```python
from build123d import *

# Parameters (mm, degrees)
SKETCH1_R           = 10
BOSS_EXTRUDE1_DEPTH = 60
SKETCH2_R           = 7.5
BOSS_EXTRUDE2_DEPTH = 30
CHAMFER2_SIZE       = 5
SKETCH3_R           = 7.5
BOSS_EXTRUDE3_DEPTH = 20
CHAMFER3_SIZE       = 4
CHAMFER3_SIZE2      = 4.76701437
SKETCH5_W           = 6
SKETCH5_H           = 55
BOSS_EXTRUDE5_DEPTH = 12
SKETCH6_W           = 2.4
SKETCH6_H           = 10
BOSS_EXTRUDE6_DEPTH = 10
SKETCH13_W          = 6
SKETCH13_H          = 1
CUT_EXTRUDE2_DEPTH  = 10
SKETCH14_W          = 6
SKETCH14_H          = 1
CUT_EXTRUDE3_DEPTH  = 5
CHAMFER22_SIZE      = 0.5
CHAMFER22_SIZE_2    = 1.866025404
SKETCH17_W          = 1
SKETCH17_H          = 2.5
BOSS_EXTRUDE7_DEPTH = 0.5
FILLET1_R           = 1
FILLET2_R           = 5


with BuildPart() as part:
    # Sketch1 → Boss-Extrude1 (new body)
    with BuildSketch(Plane(origin=(0, 0, 0), x_dir=(1, 0, 0), z_dir=(0, 1, 0))):
        with Locations(Location((0, 0, 0), (0, 0, 90))):
            Circle(SKETCH1_R)
    extrude(amount=BOSS_EXTRUDE1_DEPTH)

    # Sketch2 → Boss-Extrude2 (add)
    with BuildSketch(Plane(origin=(0, 60, 0), x_dir=(1, 0, 0), z_dir=(0, 1, 0))):
        with Locations(Location((0, 0, 0), (0, 0, 270))):
            Circle(SKETCH2_R)
    extrude(amount=BOSS_EXTRUDE2_DEPTH)

    # Chamfer2
    # the kernel refuses this chamfer: 5 mm, written as the material it takes off along each edge
    with BuildSketch(Plane(origin=(0, 60, 0), x_dir=(0, 0, -1), z_dir=(1, 0, 0))) as chamfer2_piece_1_section:
        Polygon((10, -CHAMFER2_SIZE), (10 - CHAMFER2_SIZE, 0), (10, 0), align=None)
    chamfer2_piece_1 = revolve(axis=Axis((0, 60, 0), (0, 1, 0)), mode=Mode.PRIVATE)
    chamfer2_piece_1 = chamfer2_piece_1 - Plane(origin=(0, 56.238108378, 0), x_dir=(0, 0, 1), z_dir=(0, -1, 0)) * Cylinder(7.5, 40, mode=Mode.PRIVATE)
    add(chamfer2_piece_1, mode=Mode.SUBTRACT)

    # Sketch3 → Boss-Extrude3 (add)
    with BuildSketch(Plane(origin=(0, 90, 0), x_dir=(1, 0, 0), z_dir=(0, 1, 0))):
        with Locations(Location((0, 0, 0), (0, 0, 90))):
            Circle(SKETCH3_R)
    extrude(amount=BOSS_EXTRUDE3_DEPTH)

    # Chamfer3
    chamfer3_edges = [part.edges().sort_by_distance(p)[0] for p in [
        (0, 110, 7.5),
    ]]
    chamfer3_side = [part.faces().sort_by_distance(p)[0] for p in [
        (0, 110, 0),
    ]]
    chamfer(chamfer3_edges, length=CHAMFER3_SIZE, length2=CHAMFER3_SIZE2, reference=chamfer3_side[0])

    # Sketch5 → Boss-Extrude5 (add)
    with BuildSketch(Plane(origin=(0, 0, 0), x_dir=(0, 0, -1), z_dir=(1, 0, 0))):
        with Locations((0, 27.5)):
            Rectangle(SKETCH5_W, SKETCH5_H)
    extrude(amount=BOSS_EXTRUDE5_DEPTH)

    # Sketch6 → Boss-Extrude6 (add)
    with BuildSketch(Plane(origin=(0, 0, 0), x_dir=(0, 0, -1), z_dir=(1, 0, 0))):
        with Locations((0, 87.067071975)):
            Rectangle(SKETCH6_W, SKETCH6_H)
    extrude(amount=BOSS_EXTRUDE6_DEPTH)

    # Sketch13 → Cut-Extrude2 (cut)
    with BuildSketch(Plane(origin=(0, 110, 0), x_dir=(1, 0, 0), z_dir=(0, 1, 0))):
        Rectangle(SKETCH13_W, SKETCH13_H)
    extrude(amount=-CUT_EXTRUDE2_DEPTH, mode=Mode.SUBTRACT)

    # Sketch14 → Cut-Extrude3 (cut)
    with BuildSketch(Plane(origin=(0, 100, 0), x_dir=(1, 0, 0), z_dir=(0, 1, 0))):
        Rectangle(SKETCH14_W, SKETCH14_H)
    extrude(amount=-CUT_EXTRUDE3_DEPTH, mode=Mode.SUBTRACT)

    # Chamfer22
    # the kernel refuses this chamfer: 1.866025404, 0.5 mm, written as the material it takes off along each edge
    with BuildSketch(Plane(origin=(3, 110, 0.5), x_dir=(0.9905000388259552, 0.13751244702128432, 0), z_dir=(0, 0, -1)), Plane(origin=(-3, 110, -0.5), x_dir=(-0.9905000388259552, 0.13751244702128432, 0), z_dir=(0, 0, 1))) as chamfer22_piece_1:
        Polygon((CHAMFER22_SIZE * 0.990500038826, CHAMFER22_SIZE * 0.137512447021), (-CHAMFER22_SIZE_2 * 0.137512447005, CHAMFER22_SIZE_2 * 0.990500038712), (0, 0), align=None)
    extrude(amount=1, mode=Mode.SUBTRACT)

    # Sketch17 → Boss-Extrude7 (add)
    with BuildSketch(Plane(origin=(0, 0, 0.5), x_dir=(-1, 0, 0), z_dir=(0, 0, -1))):
        with Locations((0, 101.254046964)):
            Rectangle(SKETCH17_W, SKETCH17_H)
    extrude(amount=BOSS_EXTRUDE7_DEPTH)

    # Fillet1
    # the kernel refuses this fillet: 1 mm, written as the material it takes off along each edge
    with BuildSketch(Plane(origin=(-2.665063509, 102.504046964, 0), x_dir=(0, 0, 1), z_dir=(1, 0, 0))) as fillet1_piece_1:
        with BuildLine():
            CenterArc((1, 0.866025404), FILLET1_R, 180, 60)
            Line((0, 0.866025404), (-0.02, 0.866025404))
            Line((-0.02, 0.866025404), (-0.02, 0))
            Line((-0.02, 0), (0, -0.02))
            ThreePointArc((0, -0.02), (0.25, -0.02), (0.49, -0.017320508))
            Line((0.49, -0.017320508), (0.5, 0))
        make_face()
    extrude(amount=5.330127019, mode=Mode.SUBTRACT)

    # Fillet2
    fillet2_edges = [part.edges().sort_by_distance(p)[0] for p in [
        (3, 108.133974596, 0),
        (-3, 108.133974596, 0),
    ]]
    fillet(fillet2_edges, radius=FILLET2_R)


solid = part.part
```
Work out the finished part from the listing and answer in its coordinate system (mm). A direction names the side the tool comes from. Round coordinates to 2 decimals unless told otherwise and drop trailing zeros. Write each loop counter-clockwise with the first axis right and the second up, starting at its lowest first coordinate (ties: lowest second). Pieces come first, ordered by that corner, then holes. Notation, with made-up numbers: (28.5, 5) - (59.5, 5) arc R28 cw to (59.5, 40) - close; hole circle Ø8 at (3, 25). An arc over 180 degrees is marked (long way). Return JSON: item names as keys, results as strings. Group by question number.
Q1. The part is cut by section C-C on y = 9.5. Write down the section's boundary in (x, z), then the cut area to 3 significant figures.
Q2. The mould has two halves that part along Z. Classify faces 1 (the flat face through (1, 0, 0)), 2 (the flat face through (11, 27, -3)), 3 (the flat face through (11, 27, 3)), 4 (the flat face through (-1, 102, 0.5)): released by +Z, released by -Z, zero draft, split by the parting line, or undercut.
Q3. The part is cut by section A-A on y = 86. Write down the section's boundary in (x, z).
Q4. Each of these flat-tipped pins is pushed along its axis until it touches: pin 1 Ø2.5 at (x, y) = (11.5, 15.5) entering from +Z; pin 2 Ø1.9 at (y, z) = (87.5, 0) entering from +X; pin 3 Ø7.5 at (x, y) = (0, 100.5) entering from -Z; pin 4 Ø12 at (x, z) = (-1.5, 0.5) entering from -Y. Where does it stop, or does it pass through?
Q5. For faces 5 (the flat face through (0, 102, -0.5)), 6 (the flat face through (10, 87, 0)), 7 (the flat face through (9, 87, -1.2)), 8 (the flat face through (9, 87, 1.2)), determine the directions among +Z, -Z, +X, -X, +Y, -Y from which every point of the face is accessible in a straight line to the end or side of a thin tool.
Q6. The part is cut by section B-B on y = 61.5. Write down the section's boundary in (x, z), then the cut area to 3 significant figures.
Q7. Find the intervals of material crossed by L1, parallel to X at y = 20, z = 0.5; L2, parallel to Z at x = 0.25, y = 34; L3, parallel to Z at x = -5, y = 88, in increasing order.
Solved:
{
 "1": {"outline": "(9.54, -3) - (12, -3) - (12, 3) - (9.54, 3) arc R10 ccw (long way) to start", "area": "327 mm²"},
 "2": {"face 1": "zero draft", "face 2": "released by -Z", "face 3": "released by +Z", "face 4": "undercut"},
 "3": {"outline": "(7.4, -1.2) - (10, -1.2) - (10, 1.2) - (7.4, 1.2) arc R7.5 ccw (long way) to start"},
 "4": {"pin 1": "z = 3", "pin 2": "x = 10", "pin 3": "z = -7.5", "pin 4": "y = 0"},
 "5": {"face 5": "+Y", "face 6": "+Z, -Z, +X, +Y", "face 7": "-Z, +X, +Y", "face 8": "+Z, +X, +Y"},
 "6": {"outline": "circle Ø15 at (0, 0)", "area": "177 mm²"},
 "7": {"L1": "-9.99 to 12", "L2": "-10 to 10", "L3": "-5.59 to 5.59"}
}
